Read the model definition and answer for the solid it produces. Units are mm, in the model's axes. Face numbers are marked on the shaded views. A direction names the side the tool comes from. Coordinates: 2 decimals unless noted, no trailing zeros. Order: outer loops, then holes, each group sorted by start corner. A loop starts at its lowest first (then second) coordinate and runs counter-clockwise, first axis right, second up.
Autodesk Inventor part; units mm, degrees
ref_plane "YZ Plane" through (0, 0, 0) normal (1, 0, 0) x (0, 1, 0)
ref_plane "XZ Plane" through (0, 0, 0) normal (0, 1, 0) x (-1, 0, 0)
ref_plane "XY Plane" through (0, 0, 0) normal (0, 0, 1) x (1, 0, 0)
sketch "スケッチ1" plane through (0, 0, 0) normal (0, 1, 0) x (-1, 0, 0)
  line L0 (-12.5, -15) -> (12.5, -15)
  line L1 (12.5, -15) -> (12.5, 15)
  line L2 (12.5, 15) -> (-12.5, 15)
  line L3 (-12.5, 15) -> (-12.5, -15)
  line L4 (-12.5, -15) -> (12.5, 15) construction
  line L5 (12.5, -15) -> (-12.5, 15) construction
  point P0 (0, 0)
  dimension "d0" = 25
  dimension "d1" = 30
extrude "押し出し1" add sketch "スケッチ1" along normal blind 25
sketch "スケッチ2" plane through (0, 0, 0) normal (0, -1, 0) x (1, 0, 0)
  line L0 (12.5, 15) -> (12.5, -15)
  line L1 (12.5, -10.25) -> (-8, -10.25)
  line L2 (-8, -10.25) -> (-8, 10.25)
  line L3 (-8, 10.25) -> (12.5, 10.25)
  line L4 (12.5, 10.25) -> (12.5, -10.25)
  line L5 (12.5, -15) -> (-12.5, -15)
  point P0 (0, 0)
  point P1 (12.5, 10.25)
  dimension "d4" = 20.5
  dimension "d5" = 20.5
  dimension "d22" = 10.25
extrude "押し出し2" cut sketch "スケッチ2" against normal blind 20
sketch "スケッチ4" plane through (12.5, 0, -15) normal (0, 0, -1) x (-1, 0, 0)
  line L0 (0, 0) -> (25, 0)
  line L1 (0, 0) -> (0, 25)
  point P0 (12.5, 0)
  point P1 (10.25, 7)
  dimension "d12" = 7
  dimension "d13" = 10.25
hole "穴1" at (2.25, 7, -15) direction (0, 0, 1) diameter 6 end through all
sketch "スケッチ5" plane through (0, 20, 0) normal (0, -1, 0) x (1, 0, 0)
  circle A0 centre (-2, 0) radius 6.75
  line L0 (12.5, 10.25) -> (12.5, -10.25)
  line L1 (-8, 10.25) -> (12.5, 10.25)
  line L2 (-12.5, -15) -> (-12.5, 15)
  point P0 (0, 0)
  dimension "d24" = 13.5
  dimension "d26" = 10.25
  dimension "d49" = 10.5
extrude "押し出し4" cut sketch "スケッチ5" against normal blind 4
sketch "スケッチ6" plane through (0, 25, 0) normal (0, 1, 0) x (1, 0, 0)
  line L0 (-12.5, 15) -> (-12.5, -15)
  line L1 (12.5, -15) -> (12.5, -10.25)
  line L2 (-12.5, 15) -> (12.5, 15)
  line L3 (12.5, 15) -> (12.5, -15)
  line L4 (12.5, -15) -> (-12.5, -15)
  line L5 (-12.5, -15) -> (-12.5, 15)
  point P0 (0, 0)
extrude "押し出し5" add sketch "スケッチ6" along normal blind 11
sketch "スケッチ8" plane through (-12.5, 0, -15) normal (-1, 0, 0) x (0, 0, 1)
  point P0 (15, 0)
sketch "スケッチ9" plane through (-12.5, 0, -15) normal (-1, 0, 0) x (0, 0, 1)
  line L0 (4, 34) -> (26, 34)
  line L1 (26, 34) -> (26, 25)
  line L2 (26, 25) -> (4, 25)
  line L3 (4, 25) -> (4, 34)
  line L4 (0, 36) -> (30, 36)
  point P0 (15, 0)
  dimension "d37" = 22
  dimension "d38" = 9
  dimension "d39" = 2
  dimension "d40" = 11
extrude "押し出し7" cut sketch "スケッチ9" against normal blind 22
sketch "スケッチ10" plane through (-12.5, 0, -15) normal (-1, 0, 0) x (0, 0, 1)
  line L0 (7.5, 36) -> (22.5, 36)
  line L1 (22.5, 36) -> (22.5, 34)
  line L2 (22.5, 34) -> (7.5, 34)
  line L3 (7.5, 34) -> (7.5, 36)
  line L4 (0, 36) -> (30, 36)
  point P0 (15, 0)
  dimension "d43" = 15
  dimension "d44" = 2
  dimension "d45" = 0
  dimension "d46" = 7.5
extrude "押し出し8" cut sketch "スケッチ10" against normal blind 19
sketch "スケッチ12" plane through (0, 20, 0) normal (0, -1, 0) x (1, 0, 0)
  circle A0 centre (-2, 0) radius 6.75
  line L0 (-2, 6.75) -> (-2, -6.75)
  line L1 (-2, -6.75) -> (8, -6.75)
  line L2 (8, -6.75) -> (8, 6.75)
  line L3 (8, 6.75) -> (-2, 6.75)
  point P0 (0, 0)
  dimension "d50" = 10
extrude "押し出し9" cut sketch "スケッチ12" against normal blind 3 contours A0 L3 L2 L1
fillet "フィレット3" radius 2 12 edges at (0, 36, -15) (-3, 36, -7.5) (-12.5, 36, -11.25) (6.5, 36, 0) (-3, 36, 7.5) (0, 36, 15) (-12.5, 36, 11.25) (12.5, 36, 0) (12.5, 18, -15) (12.5, 18, 15) (-12.5, 18, 15) (-12.5, 18, -15)
properties part number "baseA"
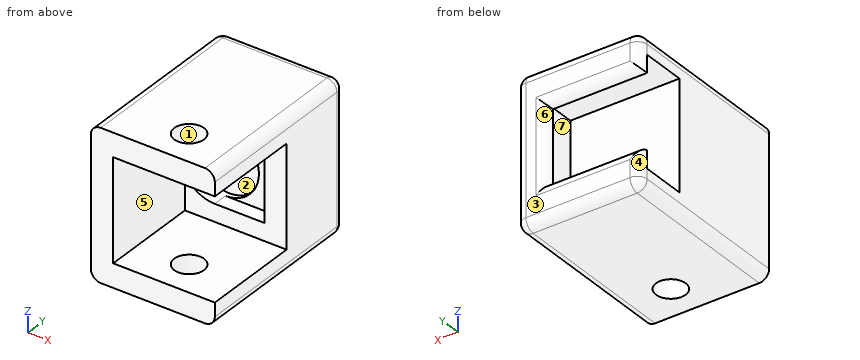
Q1. Which of the six approach directions +Z, -Z, +X, -X, +Y, -Y give full straight-line access (tool end or side, diameter ignored) to the marked faces 5, 6 and 7?
Q2. Straight lines are drawn through the part: L1, parallel to Y at x = 7.25, z = -9.5; L2, parallel to Z at x = 8.5, y = 4; L3, parallel to Z at x = -2, y = 21.55. For each, find the intervals that lie inside material, in ascending order.
Q3. The part is cut by section B-B, the plane y = 7. Determine the outline of the cut face in (x, z).
Q4. Determine the mould class of the marked faces 1, 2, 3 and 4 for opening direction X: +X half, -X half, draft (parallel to the pull), parting line (faces both ways), or undercut.
Q5. The part is cut by section A-A, the plane z = 11.5. Determine the outline of the cut face in (x, y), then the cut area to 3 significant figures.
Q6. Each of these flat-tipped pins is pushed along its axis until it touches: P1, Ø3.5, axis at x = 2.25, y = 7, coming from the -Z side; P2, Ø4.5, axis at y = 29, z = 3, coming from the -X side; P3, Ø4, axis at y = 19.5, z = -7.5, coming from the +X side; P4, Ø6.5, axis at x = -1, z = 5.5, coming from the -Y side. Where does it stop, or does it pass through?
Q7. The part is cut by section D-D, the plane y = 14. Determine the outline of the cut face in (x, z), then the cut area to 3 significant figures.
Computed values:
1. face 5: +X, -Y
1. face 6: -X, +Y
1. face 7: -X
2. L1: y = 20 to 25, 34 to 36
2. L2: z = -15 to -10.25, 10.25 to 15
2. L3: z = -15 to -6.75, 6.75 to 15
3. outline: (-12.5, -13) arc R2 ccw to (-10.5, -15) - (-0.75, -15) - (-0.75, -10.25) - (-8, -10.25) - (-8, 10.25) - (-0.75, 10.25) - (-0.75, 15) - (-10.5, 15) arc R2 ccw to (-12.5, 13) - close; (5.25, -15) - (10.5, -15) arc R2 ccw to (12.5, -13) - (12.5, -10.25) - (5.25, -10.25) - close; (5.25, 10.25) - (12.5, 10.25) - (12.5, 13) arc R2 ccw to (10.5, 15) - (5.25, 15) - close
4. face 1: undercut
4. face 2: undercut
4. face 3: draft
4. face 4: -X half
5. outline: (-12.5, 0) - (12.5, 0) - (12.5, 34) arc R2 ccw to (10.5, 36) - (-10.5, 36) arc R2 ccw to (-12.5, 34) - close; hole circle Ø6 at (2.25, 7)
5. area: 870 mm2
6. P1: passes through
6. P2: stops at x = 9.5
6. P3: stops at x = 12.5
6. P4: stops at y = 20
7. outline: (-12.5, -13) arc R2 ccw to (-10.5, -15) - (10.5, -15) arc R2 ccw to (12.5, -13) - (12.5, -10.25) - (-8, -10.25) - (-8, 10.25) - (12.5, 10.25) - (12.5, 13) arc R2 ccw to (10.5, 15) - (-10.5, 15) arc R2 ccw to (-12.5, 13) - close
7. area: 326 mm2
